```python
from build123d import *

# Parameters (mm, degrees)
SKETCH1_R               = 1.75
BOSS_EXTRUDE1_DEPTH     = 8
CUT_EXTRUDE1_DEPTH      = 48.010637094
CUT_EXTRUDE1_DEPTH_BACK = 48.010637094


with BuildPart() as part:
    # Sketch1 → Boss-Extrude1 (new body)
    with BuildSketch(Plane.XY):
        with BuildLine():
            Line((0, -39), (0, -37))
            ThreePointArc((0, -37), (22.640040384, -18.053217417), (7.979565739, 7.571428571))
            ThreePointArc((7.979565739, 7.571428571), (10.106574946, -4.342481187), (0, -11))
            ThreePointArc((0, -11), (-11, 0), (0, 11))
            ThreePointArc((0, 11), (25, -14), (0, -39))
        make_face()
        with Locations((0, 7.5)):
            Circle(SKETCH1_R, mode=Mode.SUBTRACT)
        with Locations((-7.5, 0)):
            Circle(SKETCH1_R, mode=Mode.SUBTRACT)
        with Locations((0, -7.5)):
            Circle(SKETCH1_R, mode=Mode.SUBTRACT)
        with Locations((7.5, 0)):
            Circle(SKETCH1_R, mode=Mode.SUBTRACT)
    extrude(amount=BOSS_EXTRUDE1_DEPTH)

    # Sketch2 → Cut-Extrude1 (cut, two sides: drawn at the far end of the back side and taken through both)
    with BuildSketch(Plane(origin=(0, 0, 0), x_dir=(-1, 0, 0), z_dir=(0, 0, -1)).offset(-CUT_EXTRUDE1_DEPTH_BACK)):
        Polygon((9.192388155, -8.485281374), (7.071067812, -6.363961031), (6.363961031, -7.071067812), (8.485281374, -9.192388155), align=None)
    extrude(amount=CUT_EXTRUDE1_DEPTH + CUT_EXTRUDE1_DEPTH_BACK, mode=Mode.SUBTRACT)


solid = part.part
```
Design review of the part built by this model. Coordinates are the model's own, in mm. A direction names the side the tool comes from. Coordinates: 2 decimals unless noted, no trailing zeros. Order: outer loops, then holes, each group sorted by start corner. A loop starts at its lowest first (then second) coordinate and runs counter-clockwise, first axis right, second up. Notation, with made-up numbers: (16, 16.5) -> (39, 16.5) arc R25 cw to (39, 47.5) -> close; hole circle Ø6 at (26, 67.5). An arc over 180 degrees is marked (long way). One line per item, written item: value. Start each with the question number.
Q1. For probe 1 along Y at (x, z) = (-0.5, 1.75); probe 2 along X at (y, z) = (1, 6.5); probe 3 along X at (y, z) = (-6, 3.5), list the stretches that pass through material, from the lowest coordinate up.
Q2. Take a section at B-B, the plane x = 11.5. State the section outline as (y, z) points.
Q3. Take a section at A-A, the plane y = 0. State the section outline as (x, z) points, then the cut area to 3 significant figures.
Q4. Take a section at D-D, the plane y = -14. State the section outline as (x, z) points, then the cut area to 3 significant figures.
Q5. Insertion check: pin 1 Ø1 at (x, z) = (10, 2) entering from -Y; pin 2 Ø2 at (x, y) = (7.5, 0) entering from +Z; pin 3 Ø1.5 at (x, z) = (4, 3) entering from +Y; pin 4 Ø4 at (x, z) = (20, 5) entering from -Y. Each pin has a flat end and moves straight along its axis. Give the tip position at first contact, or say it passes through.
Q6. Mouldability with a two-part tool opening along X and no side actions: class faces 1 (the cylindrical face through (-5.831, 0.526, 3.944)), 2 (the flat face through (0, -38, 4)), 3 (the cylindrical face through (24.994, -13.45, 3.944)) as pulls with the +X half, pulls with the -X half, needs draft (parallel to the pull), parting line crosses it, or undercut.
Q7. Tool access review of faces 4 (the flat face through (6, -5, 0)), 5 (the flat face through (-7.605, -6.898, 4.056)): name each direction out of +Z, -Z, +X, -X, +Y, -Y from which nothing blocks a thin tool from reaching the whole face with its end or side.
Q8. Take a section at C-C, the plane z = 7. State the section outline as (x, y) points, then the cut area to 3 significant figures.
Values follow:
1. probe 1: y = -10.99 to -9.18, -5.82 to 5.82, 9.18 to 10.99
1. probe 2: x = -10.95 to -8.94, -6.06 to 6.06, 8.94 to 10.95, 17.44 to 20
1. probe 3: x = -9.22 to -0.9, 0.9 to 9.22, 21.56 to 23.69
2. outline: (-36.2, 0) -> (-33.92, 0) -> (-33.92, 8) -> (-36.2, 8) -> close; (5.92, 0) -> (8.2, 0) -> (8.2, 8) -> (5.92, 8) -> close
3. outline: (-11, 0) -> (-9.25, 0) -> (-9.25, 8) -> (-11, 8) -> close; (-5.75, 0) -> (5.75, 0) -> (5.75, 8) -> (-5.75, 8) -> close; (9.25, 0) -> (11, 0) -> (11, 8) -> (9.25, 8) -> close; (18.25, 0) -> (20.71, 0) -> (20.71, 8) -> (18.25, 8) -> close
3. area: 140 mm2
4. outline: (23, 0) -> (25, 0) -> (25, 8) -> (23, 8) -> close
4. area: 16.0 mm2
5. pin 1: stops at y = -37.12
5. pin 2: passes through
5. pin 3: stops at y = 10.79
5. pin 4: stops at y = -31.35
6. face 1: undercut
6. face 2: pulls with the -X half
6. face 3: pulls with the +X half
7. face 4: -Z, +X, -X, +Y, -Y
7. face 5: +Z, -Z
8. outline: (-8.12, -7.42) -> (-7.07, -6.36) -> (-6.36, -7.07) -> (-7.42, -8.12) arc R11 ccw to (7.98, 7.57) arc R23 cw to (0, -37) -> (0, -39) arc R25 ccw to (0, 11) arc R11 ccw to start; hole circle Ø3.5 at (-7.5, 0); hole circle Ø3.5 at (0, -7.5); hole circle Ø3.5 at (0, 7.5); hole circle Ø3.5 at (7.5, 0)
8. area: 480 mm2
